Model file for the job. Use its own axes, mm. Round coordinates to 2 decimals unless told otherwise and drop trailing zeros. Write each loop counter-clockwise with the first axis right and the second up, starting at its lowest first coordinate (ties: lowest second). Pieces come first, ordered by that corner, then holes.
Autodesk Inventor part; units mm, degrees
ref_plane "YZ Plane" through (0, 0, 0) normal (1, 0, 0) x (0, 1, 0)
ref_plane "XZ Plane" through (0, 0, 0) normal (0, 1, 0) x (-1, 0, 0)
ref_plane "XY Plane" through (0, 0, 0) normal (0, 0, 1) x (1, 0, 0)
sketch "Sketch1" plane through (0, 0, 0) normal (1, 0, 0) x (0, 1, 0)
  line L0 (0, 0) -> (76.2, 0)
  line L1 (0, 0) -> (0, 406.4)
  line L2 (0, 406.4) -> (63.5, 406.4)
  line L3 (63.5, 406.4) -> (76.2, 0)
  dimension "d0" = 76.2
  dimension "d1" = 406.4
  dimension "d2" = 63.5
extrude "Extrusion1" add sketch "Sketch1" along normal blind 1211.2625
sketch "Sketch2" plane through (0, 0, 0) normal (0, -1, 0) x (1, 0, 0)
  line L0 (0, 406.4) -> (1211.2625, 406.4)
  line L1 (1211.2625, 406.4) -> (1211.2625, 0)
  line L2 (0, 406.4) -> (0, 0)
  line L3 (1211.2625, 0) -> (1211.2625, 406.4) construction
  line L4 (1211.2625, 219.075) -> (0, 219.075) construction
  line L5 (0, 406.4) -> (1211.2625, 406.4) construction
  line L6 (1012.0312, 406.4) -> (1012.0312, 0) construction
  line L7 (0, 0) -> (1211.2625, 0) construction
  line L8 (199.2312, 406.4) -> (199.2312, 0) construction
  line L9 (605.6313, 0) -> (605.6313, 406.4) construction
  circle A0 centre (1012.0312, 219.075) radius 4.7625
  circle A1 centre (199.2312, 219.075) radius 4.7625
  dimension "d5" = 187.325
  dimension "d6" = 812.8
  dimension "d7" = 9.525
  dimension "d8" = 9.525
extrude "Extrusion2" cut sketch "Sketch2" against normal blind 38.1
equation "\"d8\" = d7"
properties part number "Coping - 4" material "Granite, Cut, Polished"
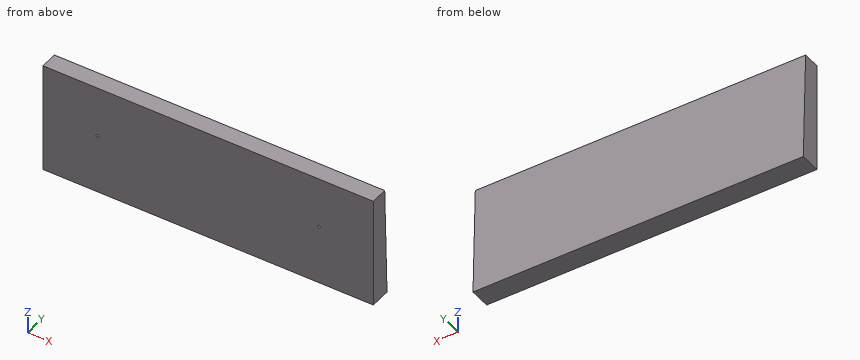
1) Wall check: probe 1 along Y at (x, z) = (915.5, 275.5); probe 2 along Y at (x, z) = (551, 120). Give the ranges that are in metal, low to high.
2) Cut at A-A on x = 950. List the corners of the cut face in (y, z), and give its area (3 significant figures).
3) Flat gauge pins, fed straight in: pin 1 Ø3 at (x, z) = (198.5, 218.5) entering from -Y; pin 2 Ø2 at (x, z) = (880.5, 197) entering from +Y (3 decimals); pin 3 Ø1.5 at (x, z) = (741.5, 213.5) entering from +Y. Where does each tip first touch, or does it go through?
4) Cut at B-B on z = 99. List the corners of the cut face in (x, y).
Result sheet:
1. probe 1: y = 0 to 67.59
1. probe 2: y = 0 to 72.45
2. outline: (0, 0) - (76.2, 0) - (63.5, 406.4) - (0, 406.4) - close
2. area: 28,400 mm2
3. pin 1: stops at y = 38.1
3. pin 2: stops at y = 70.075
3. pin 3: stops at y = 69.55
4. outline: (0, 0) - (1211.26, 0) - (1211.26, 73.11) - (0, 73.11) - close
